from build123d import *

# Parameters (mm, degrees)
SKETCH1_W                = 20.19
SKETCH1_H                = 20.19
BOSS_EXTRUDE1_DEPTH      = 2.01
SKETCH2_R                = 1.25
CUT_EXTRUDE1_DEPTH       = 2.01
FILLET1_R                = 2.85
BOSS_EXTRUDE2_DEPTH      = 9.5
SKETCH5_W                = 10.26
SKETCH5_H                = 2.578976508
CUT_EXTRUDE2_DEPTH       = 1
CUT_EXTRUDE3_REACH       = 21.19
SKETCH6_W                = 2.5
SKETCH6_H                = 2.578976508
SKETCH7_R                = 6.25
BOSS_EXTRUDE3_DEPTH      = 4.19
SKETCH8_R                = 0.73
BOSS_EXTRUDE4_DEPTH      = 8.19
BOSS_EXTRUDE4_DEPTH_BACK = 7
FILLET2_R                = 0.5
SKETCH9_R                = 1.25
SKETCH9_R_2              = 1
SKETCH9_W                = 2.5
SKETCH9_H                = 2.5
SKETCH9_W_2              = 2
SKETCH9_H_2              = 2
EXTRUDE_THIN1_DEPTH      = 6.5
SKETCH10_W               = 1.5
SKETCH10_H               = 2.01
CUT_EXTRUDE4_DEPTH       = 0.1
SKETCH12_W               = 2.01
SKETCH12_H               = 1.5
CUT_EXTRUDE5_DEPTH       = 0.1


with BuildPart() as part:
    # Sketch1 → Boss-Extrude1 (new body)
    with BuildSketch(Plane.XY):
        Rectangle(SKETCH1_W, SKETCH1_H)
    extrude(amount=BOSS_EXTRUDE1_DEPTH)

    # Sketch2 → Cut-Extrude1 (cut)
    with BuildSketch(Plane.XY.offset(2.01)):
        with Locations((-7.25, 7.25)):
            Circle(SKETCH2_R)
        with Locations((7.25, 7.25)):
            Circle(SKETCH2_R)
        with Locations((7.25, -7.25)):
            Circle(SKETCH2_R)
        with Locations((-7.25, -7.25)):
            Circle(SKETCH2_R)
    extrude(amount=-CUT_EXTRUDE1_DEPTH, mode=Mode.SUBTRACT)

    # Fillet1
    fillet1_edges = [part.edges().sort_by_distance(p)[0] for p in [
        (10.095, -10.095, 1.005),
        (-10.095, -10.095, 1.005),
        (-10.095, 10.095, 1.005),
        (10.095, 10.095, 1.005),
    ]]
    fillet(fillet1_edges, radius=FILLET1_R)

    # Sketch4 → Boss-Extrude2 (add)
    with BuildSketch(Plane.XY.offset(2.01)):
        with BuildLine():
            Line((-10.095, -2.749488254), (-10.095, 2.749488254))
            Line((-10.095, 2.749488254), (-7.633895652, 2.749488254))
            ThreePointArc((-7.633895652, 2.749488254), (-7.10515041, 2.900707677), (-6.736318268, 3.308631317))
            ThreePointArc((-6.736318268, 3.308631317), (7.505, 0), (-6.736318268, -3.308631317))
            ThreePointArc((-6.736318268, -3.308631317), (-7.10515041, -2.900707677), (-7.633895652, -2.749488254))
            Line((-7.633895652, -2.749488254), (-10.095, -2.749488254))
        make_face()
        with BuildLine():
            Line((-8.635, -1.289488254), (-8.635, 1.289488254))
            Line((-8.635, 1.289488254), (-7.633895652, 1.289488254))
            ThreePointArc((-7.633895652, 1.289488254), (-6.333182356, 1.661488034), (-5.425855287, 2.664980188))
            ThreePointArc((-5.425855287, 2.664980188), (6.045, 0), (-5.425855287, -2.664980188))
            ThreePointArc((-5.425855287, -2.664980188), (-6.333182356, -1.661488034), (-7.633895652, -1.289488254))
            Line((-7.633895652, -1.289488254), (-8.635, -1.289488254))
        make_face(mode=Mode.SUBTRACT)
    extrude(amount=BOSS_EXTRUDE2_DEPTH)

    # Sketch5 → Cut-Extrude2 (cut)
    with BuildSketch(Plane.ZY.offset(10.095)):
        with Locations((5.13, 0)):
            Rectangle(SKETCH5_W, SKETCH5_H)
    extrude(amount=-CUT_EXTRUDE2_DEPTH, mode=Mode.SUBTRACT)

    # Sketch6 → Cut-Extrude3 (cut, up to next)
    with BuildSketch(Plane.ZY.offset(9.095), mode=Mode.PRIVATE) as cut_extrude3_sk1:
        with Locations((9.01, 0)):
            Rectangle(SKETCH6_W, SKETCH6_H)
    cut_extrude3_tool1 = extrude(cut_extrude3_sk1.sketch, amount=-CUT_EXTRUDE3_REACH, mode=Mode.PRIVATE) & part.part
    add(cut_extrude3_tool1.solids().sort_by_distance((-9.095, 0, 9.01))[0], mode=Mode.SUBTRACT)

    # Sketch7 → Boss-Extrude3 (add)
    with BuildSketch(Plane(origin=(0, 0, 0), x_dir=(-1, 0, 0), z_dir=(0, 0, -1))):
        Circle(SKETCH7_R)
    extrude(amount=BOSS_EXTRUDE3_DEPTH)

    # Sketch8 → Boss-Extrude4 (add, two sides)
    with BuildSketch(Plane.XY.offset(2.01)) as boss_extrude4_sk:
        Circle(SKETCH8_R)
        with Locations((3.445, 0)):
            Circle(SKETCH8_R)
        with Locations((1.7225, 2.983457516)):
            Circle(SKETCH8_R)
        with Locations((-1.7225, 2.983457516)):
            Circle(SKETCH8_R)
        with Locations((1.7225, -2.983457516)):
            Circle(SKETCH8_R)
        with Locations((-1.7225, -2.983457516)):
            Circle(SKETCH8_R)
    extrude(amount=BOSS_EXTRUDE4_DEPTH)
    extrude(boss_extrude4_sk.sketch, amount=-BOSS_EXTRUDE4_DEPTH_BACK)

    # Fillet2
    fillet2_edges = [part.edges().sort_by_distance(p)[0] for p in [
        (-0.73, 0, 10.2),
        (2.715, 0, 10.2),
        (0.9925, 2.983457516, 10.2),
        (-2.4525, 2.983457516, 10.2),
        (0.9925, -2.983457516, 10.2),
        (-2.4525, -2.983457516, 10.2),
    ]]
    fillet(fillet2_edges, radius=FILLET2_R)

    # Sketch9 → Extrude-Thin1 (add)
    with BuildSketch(Plane(origin=(0, 0, -4.19), x_dir=(-1, 0, 0), z_dir=(0, 0, -1))):
        with Locations((-1.7225, 2.983457516)):
            Circle(SKETCH9_R)
        with Locations((-1.7225, 2.983457516)):
            Circle(SKETCH9_R_2, mode=Mode.SUBTRACT)
        Circle(SKETCH9_R)
        Circle(SKETCH9_R_2, mode=Mode.SUBTRACT)
        with Locations((-3.445, 0)):
            Circle(SKETCH9_R)
        with Locations((-3.445, 0)):
            Circle(SKETCH9_R_2, mode=Mode.SUBTRACT)
        with Locations((-1.7225, -2.983457516)):
            Circle(SKETCH9_R)
        with Locations((-1.7225, -2.983457516)):
            Circle(SKETCH9_R_2, mode=Mode.SUBTRACT)
        with Locations((1.7225, 2.983457516)):
            Rectangle(SKETCH9_W, SKETCH9_H)
        with Locations((1.7225, 2.983457516)):
            Rectangle(SKETCH9_W_2, SKETCH9_H_2, mode=Mode.SUBTRACT)
        with Locations((1.7225, -2.983457516)):
            Rectangle(SKETCH9_W, SKETCH9_H)
        with Locations((1.7225, -2.983457516)):
            Rectangle(SKETCH9_W_2, SKETCH9_H_2, mode=Mode.SUBTRACT)
    extrude(amount=EXTRUDE_THIN1_DEPTH)

    # Sketch10 → Cut-Extrude4 (cut)
    with BuildSketch(Plane(origin=(0, 10.095, 0), x_dir=(1, 0, 0), z_dir=(0, 1, 0))):
        with Locations((0, -1.005)):
            Rectangle(SKETCH10_W, SKETCH10_H)
    extrude(amount=-CUT_EXTRUDE4_DEPTH, mode=Mode.SUBTRACT)

    # Sketch12 → Cut-Extrude5 (cut)
    with BuildSketch(Plane(origin=(10.095, 0, 0), x_dir=(0, 0, -1), z_dir=(1, 0, 0))):
        with Locations((-1.005, 0)):
            Rectangle(SKETCH12_W, SKETCH12_H)
    extrude(amount=-CUT_EXTRUDE5_DEPTH, mode=Mode.SUBTRACT)


solid = part.part
Input: part model. Units: mm. Frame: model coordinates. A direction names the side the tool comes from. Coordinates: 2 decimals unless noted, no trailing zeros. Order: outer loops, then holes, each group sorted by start corner. A loop starts at its lowest first (then second) coordinate and runs counter-clockwise, first axis right, second up.
1. Access query for faces 1 (the flat face through (-9, -2.749, 7)), 2 (the cylindrical face through (7.5, 0.3, 6.7)), 3 (the cylindrical face through (0.769, 3.284, -7.395)). Directions: +Z, -Z, +X, -X, +Y, -Y. A direction counts if a zero-diameter tool reaches every point of the face in a straight line with its end or side. Return the directions, or none.
Checked values:
face 1: +Z, -X, -Y
face 2: +Z
face 3: -Z
2. Cut plane A-A, the plane z = 6.5. Return loops of the section in (x, y) (1 decimal).
Checked values:
outline: (-10.1, -2.7) - (-7.6, -2.7) arc R1 cw to (-6.7, -3.3) arc R7.5 ccw (long way) to (-6.7, 3.3) arc R1 cw to (-7.6, 2.7) - (-10.1, 2.7) - (-10.1, 1.3) - (-9.1, 1.3) - (-9.1, -1.3) - (-10.1, -1.3) - close; circle Ø1.5 at (-1.7, -3); circle Ø1.5 at (-1.7, 3); circle Ø1.5 at (0, 0); circle Ø1.5 at (1.7, -3); circle Ø1.5 at (1.7, 3); circle Ø1.5 at (3.4, 0); hole (-8.6, -1.3) - (-7.6, -1.3) arc R2.5 cw to (-5.4, -2.7) arc R6 ccw (long way) to (-5.4, 2.7) arc R2.5 cw to (-7.6, 1.3) - (-8.6, 1.3) - close
3. Draft query along Y for faces 4 (the cylindrical face through (0.7, 0.2, -4.6)), 5 (the flat face through (-4, 10.095, 1)), 6 (the flat face through (7, -4, 2.01)). Return one class per face: +Y half, -Y half, draft (parallel to the pull), parting line (faces both ways), or undercut.
Checked values:
face 4: undercut
face 5: +Y half
face 6: draft
4. Contact query for flat-ended pins moving along their axis: P1, Ø2, axis at x = 7.25, y = 7.25, coming from the -Z side; P2, Ø1.6, axis at y = 3, z = -8.5, coming from the -X side; P3, Ø1.2, axis at x = -9, z = 7, coming from the -Y side; P4, Ø5, axis at x = 7, z = 7.5, coming from the +Y side. Output: stop coordinate, or through.
Checked values:
P1: passes through
P2: stops at x = -2.97
P3: stops at y = -2.75
P4: stops at y = 6.01
5. Cut plane C-C, the plane z = -1.75. Return loops of the section in (x, y).
Checked values:
outline: circle Ø12.5 at (0, 0)
6. Ray query, line 1 along Y through (x, z) = (0, 9) (3 decimals); line 2 along Y through (x, z) = (-8, 3.5); line 3 along Y through (x, z) = (0, -8.5). Return the intervals inside material, ascending.
Checked values:
line 1: y = -7.505 to -6.045, -0.73 to 0.73, 6.045 to 7.505
line 2: y = -2.75 to -1.29, 1.29 to 2.75
line 3: y = -1.25 to -1, 1 to 1.25
7. Cut plane D-D, the plane x = 6.75. Return loops of the section in (y, z) (3 decimals), plus the area to 3 significant figures.
Checked values:
outline: (-10.095, 0) - (-8.396, 0) - (-8.396, 2.01) - (-10.095, 2.01) - close; (-6.104, 0) - (6.104, 0) - (6.104, 2.01) - (3.281, 2.01) - (3.281, 11.51) - (-3.281, 11.51) - (-3.281, 2.01) - (-6.104, 2.01) - close; (8.396, 0) - (10.095, 0) - (10.095, 2.01) - (8.396, 2.01) - close
area: 93.7 mm2
8. Cut plane B-B, the plane x = -8. Return loops of the section in (y, z), plus the area to 3 significant figures.
Checked values:
outline: (-9.99, 0) - (-8.25, 0) - (-8.25, 2.01) - (-9.99, 2.01) - close; (-6.25, 0) - (6.25, 0) - (6.25, 2.01) - (2.75, 2.01) - (2.75, 11.51) - (1.29, 11.51) - (1.29, 2.01) - (-1.29, 2.01) - (-1.29, 11.51) - (-2.75, 11.51) - (-2.75, 2.01) - (-6.25, 2.01) - close; (8.25, 0) - (9.99, 0) - (9.99, 2.01) - (8.25, 2.01) - close
area: 59.9 mm2
